Can you work these out from the model? Positions are in its coordinate system, mm. Face numbers are marked on the shaded views. A direction names the side the tool comes from. Give positions to 0.01 mm unless a question says otherwise; leave off trailing zeros. Loops run counter-clockwise (first coordinate to the right, second up) from the corner with the lowest first, then second, coordinate; pieces in that order, holes last. Notation, with made-up numbers: (57, 88.5) -> (87, 88.5) arc R22 ccw to (87, 100.5) -> close; hole circle Ø9 at (80, 3.25). An arc over 180 degrees is marked (long way). Return JSON: item names as keys, results as strings. Group by question number.
Q1. Suppose I cut it at B-B, the plane z = -2. Please give me the cut outline in (x, y).
Q2. I need wall thicknesses on line 1 along Z through (x, y) = (-11, 2.45); line 2 along Z through (x, y) = (-1.25, 11); line 3 along Z through (x, y) = (-11, 5.5). Which ranges of each line are inside material? Lowest first, please. Write a range as [from, to].
Q3. Which directions (+Z, -Z, +X, -X, +Y, -Y) give clear straight access to the entire face, cutting with the end or side of a thin tool? Please do the marked faces 1 and 2.
Q4. Will these pins go through, and if not, where does the flat tip stop? pin 1 (1.8 mm diameter, centred on y = 12.5, z = 0, fed in from -X); pin 2 (5 mm diameter, centred on x = -12.5, y = 6.5, fed in from +Z); pin 3 (4 mm diameter, centred on x = -11, z = -4, fed in from +Y).
Q5. Suppose I cut it at A-A, the plane z = -4. Please give me the cut outline in (x, y), and give its area (3 significant figures).
Q6. Thinking about a two-plate mould opening in X: for the marked faces 3, 4, 5 and 6, which applies, pulls with the +X half, pulls with the -X half, needs draft (parallel to the pull), parting line crosses it, or undercut?
Q7. Suppose I cut it at C-C, the plane y = 11. Count the separate pieces of the cut face and the enclosed holes in it, and give its area (3 significant figures).
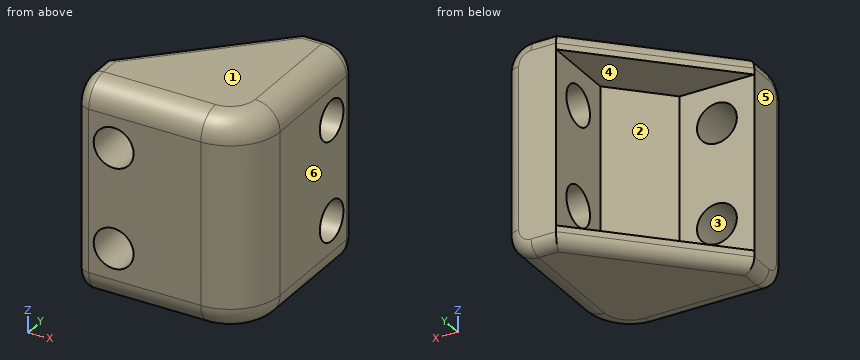
Autodesk Inventor part; units mm, degrees
ref_plane "YZ Plane" through (0, 0, 0) normal (1, 0, 0) x (0, 1, 0)
ref_plane "XZ Plane" through (0, 0, 0) normal (0, 1, 0) x (-1, 0, 0)
ref_plane "XY Plane" through (0, 0, 0) normal (0, 0, 1) x (1, 0, 0)
sketch "スケッチ1" plane through (0, 0, 0) normal (0, 0, 1) x (1, 0, 0)
  line L0 (0, 0) -> (-14, 0)
  line L1 (-14, 0) -> (-14, 14)
  line L2 (-14, 14) -> (0, 14)
  line L3 (0, 14) -> (0, 0)
  line L4 (-4, 14) -> (-14, 4)
  line L5 (-14, 4) -> (0, 4)
  line L6 (-4, 14) -> (-4, 0)
  line L7 (-4, 8) -> (-8, 4)
  dimension "d0" = 14
  dimension "d1" = 14
  dimension "d2" = 4
  dimension "d3" = 4
  dimension "d4" = 6
extrude "押し出し1" add sketch "スケッチ1" along normal blind 7 contours L0 L6 L5 L3 | L0 L1 L5 L6 | L5 L6 L2 L3 | L5 L7 L6
sketch "スケッチ2" plane through (0, 0, 7) normal (0, 0, 1) x (1, 0, 0)
  line L0 (-8, 4) -> (-14, 4)
  line L1 (0, 14) -> (-4, 14)
  line L2 (-14, 4) -> (-4, 14)
  line L3 (-4, 14) -> (0, 14)
  line L4 (0, 14) -> (0, 0)
  line L5 (0, 0) -> (-14, 0)
  line L6 (-14, 0) -> (-14, 4)
extrude "押し出し2" add sketch "スケッチ2" along normal blind 1.5
mirror "ミラー1" about plane through (-7, 7, 0) normal (0, 0, -1) of "押し出し1", "押し出し2"
sketch "スケッチ3" plane through (-4, 8, 7) normal (-1, 0, 0) x (0, 0, 1)
  line L0 (-14, 6) -> (0, 6)
  line L1 (-7, 6) -> (-7, 0)
  line L2 (0, 0) -> (-14, 0)
  line L3 (-14, 6) -> (-14, 0)
  line L4 (-14, 3) -> (0, 3)
  line L5 (0, 6) -> (0, -4)
  line L6 (-15.5, -8) -> (1.5, -8)
  point P0 (-7, -8)
  point P1 (-7, 3)
  point P2 (-3, 3)
  point P3 (-11, 3)
  dimension "d10" = 4
  dimension "d30" = 3
hole "穴1" at (-4, 11, -4) at (-4, 11, 4) direction (1, 0, 0) diameter 3.2 depth 20 tip angle 118
sketch "スケッチ4" plane through (-14, 4, 7) normal (0, 1, 0) x (1, 0, 0)
  line L0 (0, 14) -> (0, 0)
  line L1 (0, 7) -> (6, 7)
  line L2 (6, 14) -> (6, 0)
  line L3 (6, 0) -> (0, 0)
  line L4 (3, 0) -> (3, 14)
  line L5 (6, 14) -> (0, 14)
  point P0 (14, 7)
  point P1 (3, 7)
  point P2 (3, 3)
  point P3 (3, 11)
  dimension "d18" = 3
  dimension "d19" = 4
hole "穴2" at (-11, 4, -4) at (-11, 4, 4) direction (0, -1, 0) diameter 3.2 depth 20 tip angle 118
fillet "フィレット1" radius 4 1 edges at (0, 0, 0)
fillet "フィレット2" radius 2 6 edges at (-1.1716, 1.1716, 8.5) (0, 9, 8.5) (-9, 0, 8.5) (0, 9, -8.5) (-9, 0, -8.5) (-1.1716, 1.1716, -8.5)
fillet "フィレット3" radius 1 12 edges at (-0.5858, 14, 7.9142) (-3, 14, 8.5) (-0.5858, 14, -7.9142) (-3, 14, -8.5) (0, 14, 0) (-9, 9, 8.5) (-9, 9, -8.5) (-14, 0.5858, 7.9142) (-14, 3, 8.5) (-14, 0.5858, -7.9142) (-14, 3, -8.5) (-14, 0, 0)
properties part number "link2part3"
Ans:
{
 "1": {"outline": "(-14, 1) arc R1 ccw to (-13, 0) -> (-4, 0) arc R4 ccw to (0, 4) -> (0, 13) arc R1 ccw to (-1, 14) -> (-4, 14) -> (-4, 8) -> (-8, 4) -> (-14, 4) -> close"},
 "2": {"line 1": "z = [-8.5, -5.6], [-2.4, 2.4], [5.6, 8.5]", "line 2": "z = [-8.35, -5.6], [-2.4, 2.4], [5.6, 8.35]", "line 3": "z = [-8.5, -7], [7, 8.5]"},
 "3": {"face 1": "+Z, +X, -X, +Y, -Y", "face 2": "-X, +Y"},
 "4": {"pin 1": "stops at x = -4", "pin 2": "stops at z = 8.5", "pin 3": "stops at y = 4"},
 "5": {"outline": "(-14, 1) arc R1 ccw to (-13, 0) -> (-12.6, 0) -> (-12.6, 4) -> (-14, 4) -> close; (-9.4, 0) -> (-4, 0) arc R4 ccw to (0, 4) -> (0, 9.4) -> (-4, 9.4) -> (-4, 8) -> (-8, 4) -> (-9.4, 4) -> close; (-4, 12.6) -> (0, 12.6) -> (0, 13) arc R1 ccw to (-1, 14) -> (-4, 14) -> close", "area": "74.5 mm^2"},
 "6": {"face 3": "undercut", "face 4": "needs draft", "face 5": "pulls with the -X half", "face 6": "pulls with the +X half"},
 "7": {"separate pieces": "3", "enclosed holes": "0", "area": "49.1 mm^2"}
}
